Geometry check sheet. Reference: the model listing, model coordinates, mm. A direction names the side the tool comes from. Give positions to 0.01 mm unless a question says otherwise; leave off trailing zeros. Write each loop counter-clockwise with the first axis right and the second up, starting at its lowest first coordinate (ties: lowest second). Pieces come first, ordered by that corner, then holes. Notation, with made-up numbers: M 82,85.5 L 95,85.5 A26 ccw 95,115.5 Z; hole C 38,85.25 d9. An arc over 180 degrees is marked long. Write each question's results on one line, items separated by ' | '.
```python
from build123d import *

# Parameters (mm, degrees)
BOX_W          = 10
BOX_H          = 1
BOX_DEPTH      = 2
CYLINDER_R     = 2
CYLINDER_DEPTH = 10


with BuildPart() as cube:
    # Box → Box (new body)
    with BuildSketch(Plane(origin=(-5, 0, 11.2), x_dir=(1, 0, 0), z_dir=(0, 0, 1))):
        with Locations((5, 0.5)):
            Rectangle(BOX_W, BOX_H)
    extrude(amount=BOX_DEPTH)


with BuildPart() as cut:
    # Cone → Cone (revolve)
    with BuildSketch(Plane(origin=(0, 0, 10), x_dir=(1, 0, 0), z_dir=(0, -1, 0))):
        Polygon((0, 0), (2, 0), (2.8, 2.2), (0, 2.2), align=None)
    revolve(axis=Axis((0, 0, 10), (0, 0, 1)))

    # Cut: cut Cube
    add(cube.part, mode=Mode.SUBTRACT)


with BuildPart() as fusion:
    # Cylinder → Cylinder (new body)
    with BuildSketch(Plane.XY):
        Circle(CYLINDER_R)
    extrude(amount=CYLINDER_DEPTH)

    # Fusion: union Cut
    add(cut.part)


solid = fusion.part
```
Q1. Section check B-B (z = 11.5). Enter the section's corners in (x, y).
Answer key:
outline: M -2.55,0 A2.55 ccw 2.55,0 Z; M -2.34,1 L 2.34,1 A2.55 ccw Z
Q2. Section check A-A (x = 0). Enter the section's corners in (y, z), then the cut area to 3 significant figures.
Answer key:
outline: M -2.8,12.2 L -2,10 L -2,0 L 2,0 L 2,10 L 2.8,12.2 L 1,12.2 L 1,11.2 L 0,11.2 L 0,12.2 Z | area: 49.6 mm2
Q3. Release check for a two-part mould opening along Y. For faces 1 (the face through (0, 1, 12)), 2 (the face through (0, -1, 12.2)), 3 (the face through (1, -1.9, 10.4)) record: released by +Y, released by -Y, zero draft, split by the parting line, or undercut.
Answer key:
face 1: undercut | face 2: zero draft | face 3: split by the parting line
Q4. Depth check by flat-ended pin: P1, Ø1.1, axis at x = 1, z = 12, coming from the -Y side; P2, Ø1.5, axis at x = 2, y = 0.5, coming from the +Z side; P3, Ø1.5, axis at x = 0, z = 7, coming from the -Y side; P4, Ø1, axis at x = -2, z = 10.5, coming from the +Y side. Enter the tip coordinate at first touch or a pass-through.
Answer key:
P1: stops at y = -2.76 | P2: stops at z = 12.2 | P3: stops at y = -2 | P4: stops at y = 1.65
Q5. Access from +Z, -Z, +X, -X, +Y, -Y to the whole of each face (thin tool, end or side, straight path). Record for faces 4 (the face through (0, 2, 12.2)), 5 (the face through (0, 0.5, 11.2)), 6 (the face through (0, -2, 5)).
Answer key:
face 4: +Z, +X, -X, +Y, -Y | face 5: +Z, +X, -X | face 6: -Z
Q6. Material ranges on probe 1 along Z at (x, y) = (0.55, 0.8); probe 2 along Y at (x, z) = (-1.85, 11.5); probe 3 along X at (y, z) = (0.5, 6.25), recorded low to high. Write a range as [from, to].
Answer key:
probe 1: z = [0, 11.2] | probe 2: y = [-1.75, 0], [1, 1.75] | probe 3: x = [-1.94, 1.94]
Q7. Section check C-C (z = 5.5). Enter the section's corners in (x, y).
Answer key:
outline: C 0,0 d4
